from build123d import *

# Parameters (mm, degrees)
SKETCH1_R           = 81
SKETCH1_R_2         = 79.6
SKETCH1_R_3         = 76.4
SKETCH1_R_4         = 22.8
SKETCH1_R_5         = 20
BOSS_EXTRUDE1_DEPTH = 2
BOSS_EXTRUDE2_START = 17
SKETCH1_3_R         = 81
SKETCH1_3_R_2       = 79.6
BOSS_EXTRUDE2_DEPTH = 17
FILLET3_R           = 1
FILLET4_R           = 1
FILLET5_R           = 3


with BuildPart() as part:
    # Sketch1 → Boss-Extrude1 (new body)
    # profile 1 of 5: a face of its own
    with BuildSketch(Plane.XY):
        Circle(SKETCH1_R)
        Circle(SKETCH1_R_2, mode=Mode.SUBTRACT)
    # profile 2 of 5: a face of its own
    with BuildSketch(Plane.XY):
        Circle(SKETCH1_R_2)
        Circle(SKETCH1_R_3, mode=Mode.SUBTRACT)
    # profile 3 of 5: a face of its own
    with BuildSketch(Plane.XY):
        Circle(SKETCH1_R_3)
        Circle(SKETCH1_R_4, mode=Mode.SUBTRACT)
    # profile 4 of 5: a face of its own
    with BuildSketch(Plane.XY):
        Circle(SKETCH1_R_4)
        Circle(SKETCH1_R_5, mode=Mode.SUBTRACT)
    # profile 5 of 5: a face of its own
    with BuildSketch(Plane.XY):
        Circle(SKETCH1_R_5)
    extrude(amount=-BOSS_EXTRUDE1_DEPTH)

    # Sketch1_3 → Boss-Extrude2 (add)
    with BuildSketch(Plane.XY.offset(BOSS_EXTRUDE2_START)):
        Circle(SKETCH1_3_R)
        Circle(SKETCH1_3_R_2, mode=Mode.SUBTRACT)
    extrude(amount=-BOSS_EXTRUDE2_DEPTH)

    # Fillet3
    fillet3_edges = [part.edges().sort_by_distance(p)[0] for p in [
        (-81, 0, -2),
    ]]
    fillet(fillet3_edges, radius=FILLET3_R)

    # Fillet4
    fillet4_edges = [part.edges().sort_by_distance(p)[0] for p in [
        (-81, 0, 17),
    ]]
    fillet(fillet4_edges, radius=FILLET4_R)

    # Fillet5
    fillet5_edges = [part.edges().sort_by_distance(p)[0] for p in [
        (-79.6, 0, 0),
    ]]
    fillet(fillet5_edges, radius=FILLET5_R)


solid = part.part
Geometry check sheet. Reference: the model listing, model coordinates, mm. Give positions to 0.01 mm unless a question says otherwise; leave off trailing zeros. Write each loop counter-clockwise with the first axis right and the second up, starting at its lowest first coordinate (ties: lowest second). Pieces come first, ordered by that corner, then holes.
1) Cross-section at B-B (z = 7). Record the boundary of the cut face in (x, y).
Values follow:
outline: circle Ø162 at (0, 0); hole circle Ø159.2 at (0, 0)
2) Release check for a two-part mould opening along X. For faces 1 (the face through (43.545, 68.3, 7.619)), 2 (the face through (-1, 1, -2)), 3 (the face through (-63.168, -48.435, 10.098)) record: released by +X, released by -X, zero draft, split by the parting line, or undercut.
Values follow:
face 1: split by the parting line
face 2: zero draft
face 3: undercut
3) Go/stop test with flat-tipped pins: pin 1 Ø3 at (x, y) = (-33, 13) entering from +Z; pin 2 Ø6 at (y, z) = (-14.5, 1) entering from +X; pin 3 Ø5 at (y, z) = (45, 8) entering from -X. Record where each tip stops, or that it passes through.
Values follow:
pin 1: stops at z = 0
pin 2: stops at x = 80.18
pin 3: stops at x = -68.95
4) Thickness scan on line 1 (Y direction, x = 0, z = 9); line 2 (Z direction, x = -34, y = -53); line 3 (Y direction, x = -42, z = 2). Record the ranges inside material, lowest first.
Values follow:
line 1: y = -81 to -79.6, 79.6 to 81
line 2: z = -2 to 0
line 3: y = -69.26 to -67.42, 67.42 to 69.26
5) Cross-section at A-A (x = 0). Record the boundary of the cut face in (y, z).
Values follow:
outline: (-81, -1) arc R1 ccw to (-80, -2) - (80, -2) arc R1 ccw to (81, -1) - (81, 16) arc R1 ccw to (80, 17) - (79.6, 17) - (79.6, 3) arc R3 cw to (76.6, 0) - (-76.6, 0) arc R3 cw to (-79.6, 3) - (-79.6, 17) - (-80, 17) arc R1 ccw to (-81, 16) - close
